Design review of the part built by this model. Coordinates are the model's own, in mm. Face numbers are marked on the shaded views. A direction names the side the tool comes from. Coordinates: 2 decimals unless noted, no trailing zeros. Order: outer loops, then holes, each group sorted by start corner. A loop starts at its lowest first (then second) coordinate and runs counter-clockwise, first axis right, second up. Notation, with made-up numbers: (79, 33) -> (83, 33) arc R34 cw to (83, 69) -> close; hole circle Ø4 at (-19, 6). An arc over 180 degrees is marked (long way). Write item = value, one per line.
```python
from build123d import *

# Parameters (mm, degrees)
SKETCH2_R          = 1.4224
CUT_EXTRUDE1_DEPTH = 2.54


with BuildPart() as part:
    # Sketch1 → Revolve1 (revolve)
    with BuildSketch(Plane(origin=(0, 0, 0), x_dir=(-1, 0, 0), z_dir=(0, 1, 0)), mode=Mode.PRIVATE) as revolve1_sk:
        Polygon((0, 0), (50.165, 0), (50.165, 2.5273), (38.227, 2.5273), (38.227, 8.509), (32.512, 8.509), (27.1145, 13.9065), (6.9088, 13.9065), (1.143, 12.5984), (1.143, 4.0005), (0, 4.0005), align=None)
    revolve(revolve1_sk.sketch.rotate(Axis((0, 0, 0), (-1, 0, 0)), 180), axis=Axis((0, 0, 0), (-1, 0, 0)))

    # Sketch2 → Cut-Extrude1 (cut)
    with BuildSketch(Plane.YZ.offset(-1.143)):
        with Locations(Location((0, 7.9375, 0), (0, 0, 270))):
            Circle(SKETCH2_R)
        with Locations(Location((-9.5885, 0, 0), (0, 0, 270))):
            Circle(SKETCH2_R)
        with Locations(Location((0, -7.9375, 0), (0, 0, 90))):
            Circle(SKETCH2_R)
        with Locations(Location((9.5885, 0, 0), (0, 0, 90))):
            Circle(SKETCH2_R)
    extrude(amount=-CUT_EXTRUDE1_DEPTH, mode=Mode.SUBTRACT)


solid = part.part
```
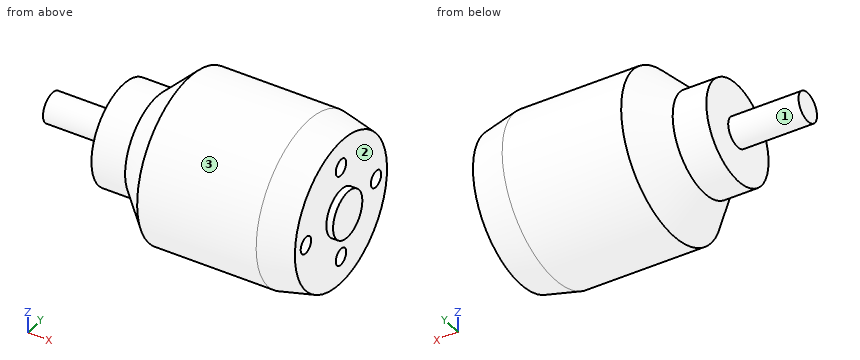
(1) For the marked faces 1, 2 and 3, list the 3-axis set-ups (+Z, -Z, +X, -X, +Y, -Y) from which the entire face can be reached by the end or side of a thin tool; tool diameter is ignored.
Report:
face_1 = -X
face_2 = +X
face_3 = +X, -X
(2) We need section A-A (y = 0). Write out the cut boundary in (x, z) (1 decimal).
Report:
outline = (-50.2, -2.5) -> (-38.2, -2.5) -> (-38.2, -8.5) -> (-32.5, -8.5) -> (-27.1, -13.9) -> (-6.9, -13.9) -> (-1.1, -12.6) -> (-1.1, -9.4) -> (-3.7, -9.4) -> (-3.7, -6.5) -> (-1.1, -6.5) -> (-1.1, -4) -> (0, -4) -> (0, 4) -> (-1.1, 4) -> (-1.1, 6.5) -> (-3.7, 6.5) -> (-3.7, 9.4) -> (-1.1, 9.4) -> (-1.1, 12.6) -> (-6.9, 13.9) -> (-27.1, 13.9) -> (-32.5, 8.5) -> (-38.2, 8.5) -> (-38.2, 2.5) -> (-50.2, 2.5) -> close
(3) Insertion check: pin 1 (3.5 mm diameter, centred on y = -9.59, z = 0, fed in from -X); pin 2 (4 mm diameter, centred on x = -26, y = 2.5, fed in from +Z); pin 3 (1 mm diameter, centred on y = 5, z = 2, fed in from +X). Each pin has a flat end and moves straight along its axis. Give the tip position at first contact, or say it passes through.
Report:
pin_1 = -38.23
pin_2 = 13.9
pin_3 = -1.14
(4) We need section C-C (x = -18). Write out the cut boundary in (y, z), and give its area (3 significant figures).
Report:
outline = circle Ø27.81 at (0, 0)
area = 608 mm²
(5) We need section B-B (z = 0). Write out the cut boundary in (x, y) (1 decimal).
Report:
outline = (-50.2, -2.5) -> (-38.2, -2.5) -> (-38.2, -8.5) -> (-32.5, -8.5) -> (-27.1, -13.9) -> (-6.9, -13.9) -> (-1.1, -12.6) -> (-1.1, -11) -> (-3.7, -11) -> (-3.7, -8.2) -> (-1.1, -8.2) -> (-1.1, -4) -> (0, -4) -> (0, 4) -> (-1.1, 4) -> (-1.1, 8.2) -> (-3.7, 8.2) -> (-3.7, 11) -> (-1.1, 11) -> (-1.1, 12.6) -> (-6.9, 13.9) -> (-27.1, 13.9) -> (-32.5, 8.5) -> (-38.2, 8.5) -> (-38.2, 2.5) -> (-50.2, 2.5) -> close
(6) For L1, parallel to Y at x = -1.85, z = 0; L2, parallel to X at y = -7.5, z = 1.75; L3, parallel to X at y = -4, z = 9.75, list the stretches that pass through material, from the lowest coordinate up.
Report:
L1 = -12.76 to -11.01, -8.17 to 8.17, 11.01 to 12.76
L2 = -38.23 to -1.14
L3 = -30.48 to -1.14
